from build123d import *

# Parameters (mm, degrees)
F0_R     = 14.2206342646
F0_R_2   = 20.3905424102
F0_R_3   = 13.8730620626
F0_R_4   = 7
F1_DEPTH = 15
F3_D     = 3.2
F5_D     = 5.25
F7_D     = 4.4
F7_DEPTH = 15
F7_TIP   = 1.3218933619


with BuildPart() as f1:
    # F0 (on Top) → F1 (new body)
    with BuildSketch(Plane.XY):
        Polygon((-80, -45), (100, -45), (100, 45), (-100, 45), (-100, 5), (-80, 5), align=None)
        with Locations((-55, -5)):
            Circle(F0_R, mode=Mode.SUBTRACT)
        with Locations((0, -5)):
            Circle(F0_R_2, mode=Mode.SUBTRACT)
        with Locations((55, -5)):
            Circle(F0_R_3, mode=Mode.SUBTRACT)
        with BuildLine():
            ThreePointArc((-86.0003137523, 35.0500990994), (-86, 35), (-86.0003137523, 34.9499009006))
            Line((-86.0003137523, 34.9499009006), (-86.0003137523, 15.0500990994))
            ThreePointArc((-86.0003137523, 15.0500990994), (-86, 15), (-86.0003137523, 14.9499009006))
            ThreePointArc((-86.0003137523, 14.9499009006), (-90.095653532, 11.0011438633), (-93.9975072002, 15.1411955542))
            Line((-93.9975072002, 15.1411955542), (-93.9999999685, 34.9994978889))
            ThreePointArc((-93.9999999685, 34.9994978889), (-90.0253010915, 38.999919981), (-86.0003137523, 35.0500990994))
        make_face(mode=Mode.SUBTRACT)
        with Locations((-30, 23)):
            Circle(F0_R_4, mode=Mode.SUBTRACT)
        with BuildLine():
            ThreePointArc((86.0107341117, 35.2928441091), (90.1465203854, 38.9973155713), (94, 35))
            Line((94, 35), (94, 15))
            ThreePointArc((94, 15), (90.1465203854, 11.0026844287), (86.0107341117, 14.7071558909))
            ThreePointArc((86.0107341117, 14.7071558909), (86, 15), (86.0107341117, 15.2928441091))
            Line((86.0107341117, 15.2928441091), (86.0107341117, 34.7071558909))
            ThreePointArc((86.0107341117, 34.7071558909), (86, 35), (86.0107341117, 35.2928441091))
        make_face(mode=Mode.SUBTRACT)
    extrude(amount=F1_DEPTH)

    # F3 (through all)
    with Locations(Plane.XY.offset(15)):
        with Locations((-74, -5), (-55, 14), (-36, -5), (-55, -24), (36, -5), (55, 14), (74, -5), (55, -24)):
            Hole(F3_D / 2)

    # F5 (through all)
    with Locations(Plane.XY.offset(15)):
        with Locations((-16.5, 24), (16.5, 24), (16.5, -34), (-16.5, -34)):
            Hole(F5_D / 2)

    # F7
    with Locations(Plane(origin=(0, 45, 0), x_dir=(-1, 0, 0), z_dir=(0, 1, 0))):
        with Locations((30, 7.5)):
            Hole(F7_D / 2, depth=F7_DEPTH)
            with Locations((0, 0, -(F7_DEPTH + F7_TIP / 2))):  # 118° drill point
                Cone(0, F7_D / 2, F7_TIP, mode=Mode.SUBTRACT)


solid = f1.part
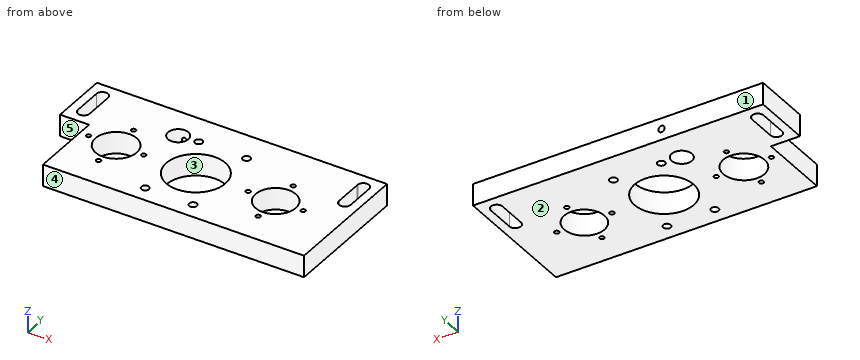
Could you check a few things on this model? Use its own coordinates, in mm. Face numbers are marked on the shaded views. A direction names the side the tool comes from. Coordinates: 2 decimals unless noted, no trailing zeros. Order: outer loops, then holes, each group sorted by start corner. A loop starts at its lowest first (then second) coordinate and runs counter-clockwise, first axis right, second up.
Q1. Will these pins go through, and if not, where does the flat tip stop? pin 1 (1.9 mm diameter, centred on x = 36, y = -5, fed in from +Z); pin 2 (8.5 mm diameter, centred on x = -16.5, y = -34, fed in from -Z).
Q2. Suppose I cut it at A-A on x = 90. Please give me the cut outline in (y, z).
Q3. Suppose I cut it at C-C on y = 18. Please give me the cut outline in (x, z), and give its area (3 significant figures).
Q4. Which directions (+Z, -Z, +X, -X, +Y, -Y) give clear straight access to the entire face, cutting with the end or side of a thin tool? Please do the marked faces 4 and 5.
Q5. Please list where these lines run through material, in increasing order: L1, parallel to Y at x = 55, z = 8; L2, parallel to Y at x = 36, z = 7.25; L3, parallel to Y at x = -36, z = 10.75.
Q6. Suppose I cut it at B-B on z = 11.75. Give the number of separate pieces and of enclosed holes in the cut face, and give its area (3 significant figures).
Q7. Suppose I cut it at D-D on x = -0.5. Please give me the cut outline in (y, z).
Q8. Thinking about a two-plate mould opening in Y: for the marked faces 1, 2 and 3, which applies, released by +Y, released by -Y, zero draft, split by the parting line, or undercut?
Answer:
1. pin 1: passes through
1. pin 2: stops at z = 0
2. outline: (-45, 0) - (11, 0) - (11, 15) - (-45, 15) - close; (39, 0) - (45, 0) - (45, 15) - (39, 15) - close
3. outline: (-100, 0) - (-94, 0) - (-94, 15) - (-100, 15) - close; (-86, 0) - (-34.9, 0) - (-34.9, 15) - (-86, 15) - close; (-25.1, 0) - (86.01, 0) - (86.01, 15) - (-25.1, 15) - close; (94, 0) - (100, 0) - (100, 15) - (94, 15) - close
3. area: 2,610 mm2
4. face 4: +Z, -Z, +X, -X, -Y
4. face 5: +Z, -Z, -X, -Y
5. L1: y = -45 to -25.6, -22.4 to -18.87, 8.87 to 12.4, 15.6 to 45
5. L2: y = -45 to -6.6, -3.4 to 45
5. L3: y = -45 to -6.6, -3.4 to 19.39, 26.61 to 45
6. separate pieces: 1
6. enclosed holes: 18
6. area: 13,700 mm2
7. outline: (-45, 0) - (-25.38, 0) - (-25.38, 15) - (-45, 15) - close; (15.38, 0) - (45, 0) - (45, 15) - (15.38, 15) - close
8. face 1: released by +Y
8. face 2: zero draft
8. face 3: undercut
